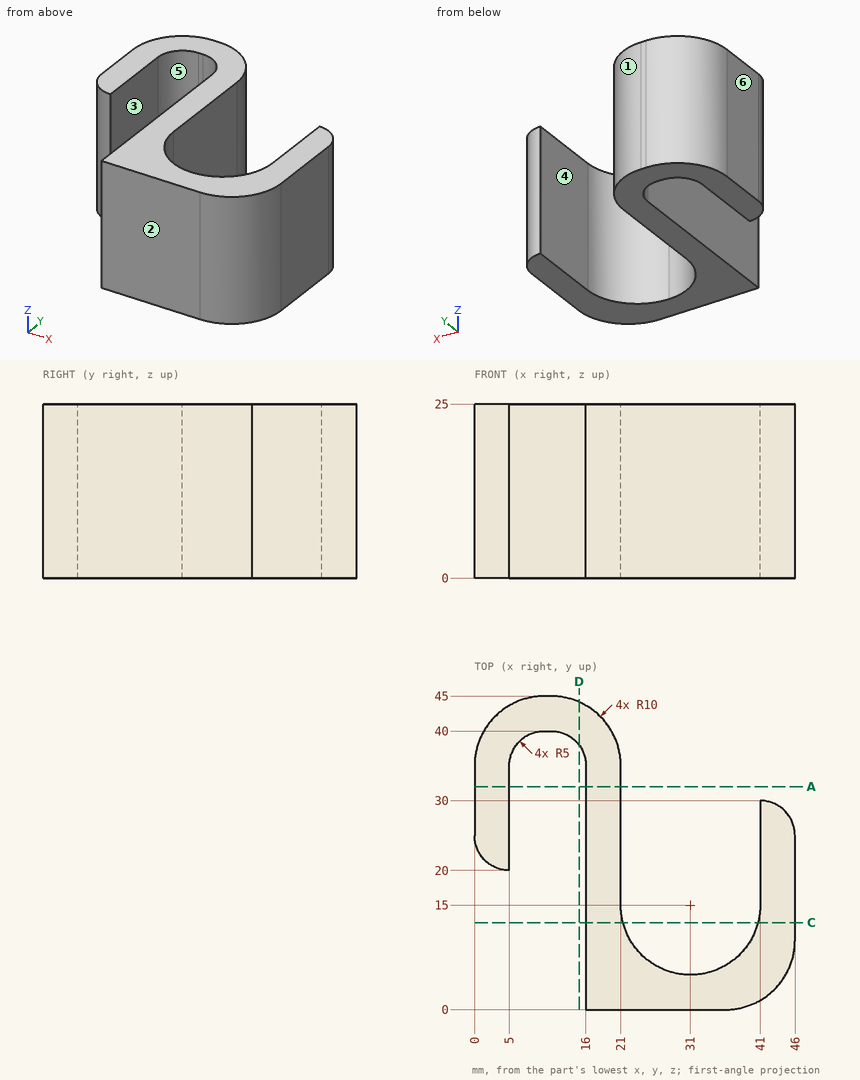
Input: dimensioned drawing with shaded views. Units: mm. Origin: part minimum x, y, z. A direction names the side the tool comes from. Round coordinates to 2 decimals unless told otherwise and drop trailing zeros. Order: outer loops, then holes, each group sorted by start corner. A loop starts at its lowest first (then second) coordinate and runs counter-clockwise, first axis right, second up. Notation, with made-up numbers: (48.5, 46.25) - (93.5, 46.25) arc R16 cw to (93.5, 71.25) - close; hole circle Ø11 at (2.25, 32). An arc over 180 degrees is marked (long way). Answer as a JSON object with one key per item and string values. Group by question number.
(1) Pin query (flat end, axial travel): P1, Ø12, axis at x = 36.5, z = 22.5, coming from the +Y side; P2, Ø2, axis at x = 37, z = 18.5, coming from the +Y side; P3, Ø0.8, axis at x = 10.5, z = 8.5, coming from the -Y side. Return the tip coordinate at first contact, or that it passes through.
(2) Draft query along X for the marked faces 1, 2 and 3. Return one class per face: released by +X, released by -X, zero draft, split by the parting line, or undercut.
(3) Material intervals for probe 1 along X at (y, z) = (32, 18.75); probe 2 along X at (y, z) = (27, 23.75); probe 3 along X at (y, z) = (22, 12.25), sorted ascending. Write a range as from..to.
(4) Cut plane A-A (y = 32). Return loops of the section in (x, z), then the cut area to 3 significant figures.
(5) Reachability of the marked faces 4, 5 and 6 from +Z, -Z, +X, -X, +Y, -Y: full face, straight path, thin tool, end or side. Return the list, or none.
(6) Cut plane D-D (x = 15). Return loops of the section in (y, z), then the cut area to 3 significant figures.
(7) Cut plane C-C (y = 12.5). Return loops of the section in (x, z).
Here are the results:
{
 "1": {"P1": "stops at y = 30", "P2": "stops at y = 7.86", "P3": "stops at y = 40"},
 "2": {"face 1": "released by +X", "face 2": "zero draft", "face 3": "undercut"},
 "3": {"probe 1": "x = 0..5, 16..21", "probe 2": "x = 0..5, 16..21, 41..45.58", "probe 3": "x = 1..5, 16..21, 41..46"},
 "4": {"outline": "(0, 0) - (5, 0) - (5, 25) - (0, 25) - close; (16, 0) - (21, 0) - (21, 25) - (16, 25) - close", "area": "250 mm^2"},
 "5": {"face 4": "+Z, -Z, +Y", "face 5": "+Z, -Z, -Y", "face 6": "+Z, -Z, -X, +Y, -Y"},
 "6": {"outline": "(38, 0) - (44.17, 0) - (44.17, 25) - (38, 25) - close", "area": "154 mm^2"},
 "7": {"outline": "(16, 0) - (21.32, 0) - (21.32, 25) - (16, 25) - close; (40.68, 0) - (46, 0) - (46, 25) - (40.68, 25) - close"}
}
